from build123d import *

# Parameters (mm, degrees)
F0_W     = 10
F0_H     = 10
F1_DEPTH = 5
F2_W     = 4
F2_H     = 4
F3_DEPTH = 15
F4_W     = 4
F4_H     = 4
F5_DEPTH = 15
F6_W     = 4
F6_H     = 4
F7_DEPTH = 15


with BuildPart() as f1:
    # F0 (on Top) → F1 (new body, symmetric)
    with BuildSketch(Plane.XY):
        Rectangle(F0_W, F0_H)
    extrude(amount=F1_DEPTH, both=True)

    # F2 (on Top) → F3 (join)
    with BuildSketch(Plane.XY):
        Rectangle(F2_W, F2_H)
    extrude(amount=F3_DEPTH)

    # F4 (on Front) → F5 (join)
    with BuildSketch(Plane.XZ):
        Rectangle(F4_W, F4_H)
    extrude(amount=F5_DEPTH)

    # F6 (on Right) → F7 (join)
    with BuildSketch(Plane.YZ):
        Rectangle(F6_W, F6_H)
    extrude(amount=F7_DEPTH)


solid = f1.part
The model under review builds one solid part; all positions refer to its coordinate system, in mm. A direction names the side the tool comes from. Round coordinates to 2 decimals unless told otherwise and drop trailing zeros. Loops run counter-clockwise (first coordinate to the right, second up) from the corner with the lowest first, then second, coordinate; pieces in that order, holes last. Notation, with made-up numbers: (-12, 5.5) -> (3, 5.5) arc R18 ccw to (3, 24.5) -> close; hole circle Ø8 at (26, -15). An arc over 180 degrees is marked (long way). Answer as CSV lines item,"result".
1) Add section B-B on y = 1. Write out the cut boundary in (x, z), plus the area to 3 significant figures.
Geometry results:
outline,"(-5, -5) -> (5, -5) -> (5, -2) -> (15, -2) -> (15, 2) -> (5, 2) -> (5, 5) -> (2, 5) -> (2, 15) -> (-2, 15) -> (-2, 5) -> (-5, 5) -> close"
area,"180 mm²"
2) Tool access review of faces 1 (the face through (0, -10, -2)), 2 (the face through (10, -2, 0)), 3 (the face through (-2, -10, 0)): name each direction out of +Z, -Z, +X, -X, +Y, -Y from which nothing blocks a thin tool from reaching the whole face with its end or side.
Geometry results:
face 1,"-Z, +X, -X, -Y"
face 2,"+Z, -Z, +X, -Y"
face 3,"+Z, -Z, -X, -Y"
3) Add section A-A on x = 1. Write out the cut boundary in (y, z).
Geometry results:
outline,"(-15, -2) -> (-5, -2) -> (-5, -5) -> (5, -5) -> (5, 5) -> (2, 5) -> (2, 15) -> (-2, 15) -> (-2, 5) -> (-5, 5) -> (-5, 2) -> (-15, 2) -> close"
4) To check wall thickness, follow line 1 along Y through (x, z) = (-0.5, -3.5); line 2 along Z through (x, y) = (7.75, 0.5). State the ranges of each line that lie inside material, in increasing order. Write a range as from..to.
Geometry results:
line 1,"y = -5..5"
line 2,"z = -2..2"
5) For P1, Ø4.5, axis at y = -11.5, z = 1, coming from the +X side; P2, Ø3, axis at x = -0.5, y = -9.5, coming from the +Z side; P3, Ø1.5, axis at x = -3, z = 0, coming from the -Y side, all flat-tipped, find the tip position at first contact; note any pin that passes through.
Geometry results:
P1,"stops at x = 2"
P2,"stops at z = 2"
P3,"stops at y = -5"
6) Add section C-C on z = -2.75. Write out the cut boundary in (x, y), plus the area to 3 significant figures.
Geometry results:
outline,"(-5, -5) -> (5, -5) -> (5, 5) -> (-5, 5) -> close"
area,"100 mm²"
7) Add section D-D on y = -7. Write out the cut boundary in (x, z).
Geometry results:
outline,"(-2, -2) -> (2, -2) -> (2, 2) -> (-2, 2) -> close"
